Autodesk Inventor part; units mm, degrees
ref_plane "YZ Plane" through (0, 0, 0) normal (1, 0, 0) x (0, 1, 0)
ref_plane "XZ Plane" through (0, 0, 0) normal (0, 1, 0) x (-1, 0, 0)
ref_plane "XY Plane" through (0, 0, 0) normal (0, 0, 1) x (1, 0, 0)
sketch "スケッチ1" plane through (0, 0, 0) normal (0, 0, 1) x (1, 0, 0)
  circle A0 centre (0, 0) radius 3.6
  dimension "d0" = 7.2
extrude "押し出し1" add sketch "スケッチ1" along normal blind 0.6
sketch "スケッチ2" plane through (0, 0, 0.6) normal (0, 0, 1) x (1, 0, 0)
  circle A0 centre (0, 0) radius 3
  dimension "d3" = 6
extrude "押し出し2" add sketch "スケッチ2" along normal blind 1.9
sketch "スケッチ3" plane through (0, 0, 2.5) normal (0, 0, 1) x (1, 0, 0)
  point P0 (0, 0)
hole "穴1" at (0, 0, 2.5) direction (0, 0, -1) diameter 3 depth 15
properties part number "ベアリング"
Source: CAD feature listing. Evaluate the final solid. Frame: model axes, mm. A direction names the side the tool comes from. Coordinates: 2 decimals unless noted, no trailing zeros. Loops run counter-clockwise (first coordinate to the right, second up) from the corner with the lowest first, then second, coordinate; pieces in that order, holes last. Notation, with made-up numbers: (26, 87) -> (44, 87) arc R28 ccw to (44, 124) -> close; hole circle Ø1 at (31, -9.5). An arc over 180 degrees is marked (long way). Answer in a Markdown table with one row per item. Add a question column.
Q1. Section C-C on z = 0.4. Return the cut outline in (x, y).
Q2. Reachability of faces 1 (the face through (1.3, -1.3, 2.5)), 2 (the face through (-1, 3, 0.6)) from +Z, -Z, +X, -X, +Y, -Y: full face, straight path, thin tool, end or side. Return the list, or none.
Q3. Ray query, line 1 along Y through (x, z) = (0, 1.7); line 2 along X through (y, z) = (1, 1.5); line 3 along Z through (x, y) = (-1.75, -2.75). Return the intervals inside material, ascending.
Q4. Section A-A on x = 0. Return the cut outline in (y, z), and give its area (3 significant figures).
Q5. Pull-direction query (Y, two-part tool) for faces 3 (the face through (-0.07, 1.5, 1.23)), 4 (the face through (3.434, -1.081, 0.296)), 5 (the face through (0, -2, 0)); classes: pulls with the +Y half, pulls with the -Y half, needs draft (parallel to the pull), parting line crosses it, or undercut.
Q6. Section D-D on x = -2.5. Return the cut outline in (y, z).
Computed values:
| question | item | result |
|---|---|---|
| 1 | outline | circle Ø7.2 at (0, 0); hole circle Ø3 at (0, 0) |
| 2 | face 1 | +Z, +X, -X, +Y, -Y |
| 2 | face 2 | +Z |
| 3 | line 1 | y = -3 to -1.5, 1.5 to 3 |
| 3 | line 2 | x = -2.83 to -1.12, 1.12 to 2.83 |
| 3 | line 3 | z = 0 to 0.6 |
| 4 | outline | (-3.6, 0) -> (-1.5, 0) -> (-1.5, 2.5) -> (-3, 2.5) -> (-3, 0.6) -> (-3.6, 0.6) -> close; (1.5, 0) -> (3.6, 0) -> (3.6, 0.6) -> (3, 0.6) -> (3, 2.5) -> (1.5, 2.5) -> close |
| 4 | area | 8.22 mm^2 |
| 5 | face 3 | undercut |
| 5 | face 4 | parting line crosses it |
| 5 | face 5 | needs draft |
| 6 | outline | (-2.59, 0) -> (2.59, 0) -> (2.59, 0.6) -> (1.66, 0.6) -> (1.66, 2.5) -> (-1.66, 2.5) -> (-1.66, 0.6) -> (-2.59, 0.6) -> close |
